from build123d import *

# Parameters (mm, degrees)
BOSS_EXTRUDE1_DEPTH = 10
SKETCH2_W           = 14
SKETCH2_H           = 4
CUT_EXTRUDE1_DEPTH  = 3
SKETCH13_R          = 1.1
CUT_EXTRUDE4_DEPTH  = 5
SKETCH14_W          = 2
SKETCH14_H          = 20
BOSS_EXTRUDE2_DEPTH = 10
BOSS_EXTRUDE3_DEPTH = 2
SKETCH17_R          = 1.1
CUT_EXTRUDE5_DEPTH  = 4
SKETCH18_W          = 10.2
SKETCH18_H          = 1
BOSS_EXTRUDE4_DEPTH = 10


with BuildPart() as part:
    # Sketch1 → Boss-Extrude1 (new, symmetric)
    with BuildSketch(Plane.XY):
        Polygon((0, 11), (0, -8), (8.2, -8), (38.2, -8), (38.2, -6), (38.2, 4), (36.2, 4), (36.2, -6), (10.2, -6), (10.2, 11), (8.2, 11), (8.2, 2), (7.2, 2), (7.2, -6), (3, -6), (3, 2), (2, 2), (2, 11), align=None)
    extrude(amount=BOSS_EXTRUDE1_DEPTH, both=True)

    # Sketch2 → Cut-Extrude1 (cut)
    with BuildSketch(Plane.ZY):
        with Locations((0, -4)):
            Rectangle(SKETCH2_W, SKETCH2_H)
    extrude(amount=-CUT_EXTRUDE1_DEPTH, mode=Mode.SUBTRACT)

    # Sketch13 → Cut-Extrude4 (cut)
    with BuildSketch(Plane.ZY):
        with Locations(Location((-5, 6.5, 0), (0, 0, 270))):
            Circle(SKETCH13_R)
        with Locations(Location((5, 6.5, 0), (0, 0, 270))):
            Circle(SKETCH13_R)
    extrude(amount=-CUT_EXTRUDE4_DEPTH, mode=Mode.SUBTRACT)

    # Sketch14 → Boss-Extrude2 (add)
    with BuildSketch(Plane.XZ.offset(8)):
        with Locations((37.2, 0)):
            Rectangle(SKETCH14_W, SKETCH14_H)
    extrude(amount=BOSS_EXTRUDE2_DEPTH)

    # Sketch15 → Boss-Extrude3 (add, symmetric)
    with BuildSketch(Plane.XY):
        Polygon((14.2, -6), (10.2, -6), (10.2, -2), align=None)
        Polygon((36.2, -6), (36.2, -2), (32.2, -6), align=None)
        Polygon((36.2, -8), (32.2, -8), (36.2, -12), align=None)
    extrude(amount=BOSS_EXTRUDE3_DEPTH, both=True)

    # Sketch17 → Cut-Extrude5 (cut)
    with BuildSketch(Plane(origin=(38.2, 0, 0), x_dir=(0, 0, -1), z_dir=(1, 0, 0))):
        with Locations((-5, -1)):
            Circle(SKETCH17_R)
        with Locations((5, -1)):
            Circle(SKETCH17_R)
        with Locations((-5, -13)):
            Circle(SKETCH17_R)
        with Locations((5, -13)):
            Circle(SKETCH17_R)
    extrude(amount=-CUT_EXTRUDE5_DEPTH, mode=Mode.SUBTRACT)

    # Sketch18 → Boss-Extrude4 (add)
    with BuildSketch(Plane(origin=(0, 11, 0), x_dir=(1, 0, 0), z_dir=(0, 1, 0))):
        with Locations((5.1, -10.5)):
            Rectangle(SKETCH18_W, SKETCH18_H)
        with Locations((5.1, 10.5)):
            Rectangle(SKETCH18_W, SKETCH18_H)
    extrude(amount=-BOSS_EXTRUDE4_DEPTH)


solid = part.part
Input: part model. Units: mm. Frame: model coordinates. A direction names the side the tool comes from. Round coordinates to 2 decimals unless told otherwise and drop trailing zeros. Order: outer loops, then holes, each group sorted by start corner. A loop starts at its lowest first (then second) coordinate and runs counter-clockwise, first axis right, second up. Notation, with made-up numbers: (-24.75, 83.5) - (-13.75, 83.5) arc R24 cw to (-13.75, 98.5) - close; hole circle Ø11 at (3.25, 8.5). An arc over 180 degrees is marked (long way). Answer as a JSON object with one key per item and string values. Group by question number.
(1) Draft query along Y for faces 6 (the face through (4, -6, 0)), 7 (the face through (8.4, 11, -0.2)), 8 (the face through (35, -9, 2)). Return one class per face: released by +Y, released by -Y, zero draft, split by the parting line, or undercut.
(2) Reachability of faces 1 (the face through (12.2, -4, 0)), 2 (the face through (36.2, -1, 0)), 3 (the face through (36.2, -13, 0)), 4 (the face through (11, -5, -2)), 5 (the face through (1, -4, 7)) from +Z, -Z, +X, -X, +Y, -Y: full face, straight path, thin tool, end or side. Return the list, or none.
(3) Cut plane B-B (z = -5). Count the separate pieces of the cut face and the enclosed holes in it, then the cut area to 3 significant figures.
(4) Cut plane A-A (y = 1.5). Return loops of the section in (x, z).
(5) Material intervals for probe 1 along Z at (x, y) = (1.6, 6.5); probe 2 along X at (y, z) = (3.25, 8.5); probe 3 along Y at (x, z) = (36.75, 5), sorted ascending. Write a range as from..to.
(6) Cut plane D-D (y = -5). Return loops of the section in (x, z).
(7) Pin query (flat end, axial travel): P1, Ø6, axis at y = 8, z = 2, coming from the +X side; P2, Ø1.5, axis at x = 1, y = -4.5, coming from the -Z side; P3, Ø10, axis at x = 28, z = 0.5, coming from the +Y side; P4, Ø1.5, axis at x = 33, y = -10, coming from the -Z side. Return the tip coordinate at first contact, or that it passes through.
(8) Cut plane C-C (y = 8.5). Return loops of the section in (x, z).
Here are the results:
{
 "1": {"face 6": "undercut", "face 7": "released by +Y", "face 8": "zero draft"},
 "2": {"face 1": "+Z, -Z, +Y", "face 2": "+Y", "face 3": "-X, -Y", "face 4": "-Z, +Y", "face 5": "-X"},
 "3": {"separate pieces": "5", "enclosed holes": "0", "area": "175 mm^2"},
 "4": {"outline": "(0, -11) - (10.2, -11) - (10.2, 11) - (0, 11) - close; (36.2, -10) - (38.2, -10) - (38.2, 10) - (36.2, 10) - close; hole (3, -10) - (7.2, -10) - (7.2, 10) - (3, 10) - close"},
 "5": {"probe 1": "z = -11..-6.1, -3.9..3.9, 6.1..11", "probe 2": "x = 0..2, 8.2..10.2, 36.2..38.2", "probe 3": "y = -18..-14.1, -11.9..-2.1, 0.1..4"},
 "6": {"outline": "(0, -10) - (3, -10) - (3, -7) - (0, -7) - close; (0, 7) - (3, 7) - (3, 10) - (0, 10) - close; (7.2, -10) - (10.2, -10) - (10.2, -2) - (13.2, -2) - (13.2, 2) - (10.2, 2) - (10.2, 10) - (7.2, 10) - close; (33.2, -2) - (36.2, -2) - (36.2, -10) - (38.2, -10) - (38.2, 10) - (36.2, 10) - (36.2, 2) - (33.2, 2) - close"},
 "7": {"P1": "stops at x = 10.2", "P2": "stops at z = -10", "P3": "stops at y = -5.2", "P4": "passes through"},
 "8": {"outline": "(0, -11) - (10.2, -11) - (10.2, 11) - (0, 11) - close; hole (2, -10) - (8.2, -10) - (8.2, 10) - (2, 10) - close"}
}
